Verification items for the finished model (mm, model axes). A direction names the side the tool comes from. Coordinates: 2 decimals unless noted, no trailing zeros. Write each loop counter-clockwise with the first axis right and the second up, starting at its lowest first coordinate (ties: lowest second). Pieces come first, ordered by that corner, then holes. Notation, with made-up numbers: M 82.25,74.5 L 119.25,74.5 A18 ccw 119.25,99.5 Z; hole C -33,38.25 d3. An arc over 180 degrees is marked long. Answer in a Markdown table with one row per item.
from build123d import *

# Parameters (mm, degrees)
BOSS_EXTRUDE2_DEPTH = 101.6
CUT_SWEEP2_START    = -8.197626231
CUT_SWEEP2_DEPTH    = 16.395252462


# Read off the part's stored shape, not the designer's step: Cut-Sweep2
with BuildPart() as part:
    # Sketch1 → Boss-Extrude2 (new, symmetric)
    with BuildSketch(Plane.XY):
        with BuildLine():
            Line((-50.8, 0), (-114.3, 0))
            Line((-114.3, 0), (-114.3, 12.7))
            Line((-114.3, 12.7), (-63.5, 12.7))
            ThreePointArc((-63.5, 12.7), (0, 64.757547823), (63.5, 12.7))
            Line((63.5, 12.7), (114.3, 12.7))
            Line((114.3, 12.7), (114.3, 0))
            Line((114.3, 0), (50.8, 0))
            ThreePointArc((50.8, 0), (0, 50.8), (-50.8, 0))
        make_face()
    extrude(amount=BOSS_EXTRUDE2_DEPTH, both=True)

    # Cut-Sweep2 outline → Cut-Sweep2 (cut)
    with BuildSketch(Plane.XY.offset(CUT_SWEEP2_START)):
        with BuildLine():
            Line((50.8, 0), (55.482597318, 0))
            add(Edge.make_bspline(
                [(55.482597318, 0), (55.479494195, 2.91415368), (55.255178285, 5.917770975), (54.175303072, 12.490458413), (53.25997788, 15.990881145), (50.641228247, 22.973888147), (48.970431753, 26.367184551), (44.847073202, 32.894857639), (42.443468127, 35.946208717), (37.009145884, 41.519887141), (34.016276899, 44.003484644), (27.57622226, 48.300783556), (24.203765584, 50.065786815), (13.800838479, 54.25746412), (6.656772523, 55.483587394), (-6.656785579, 55.483587394), (-13.800859436, 54.257459266), (-24.203789489, 50.065775387), (-27.576245764, 48.3007701), (-34.016297572, 44.003468622), (-37.009164361, 41.519870489), (-42.443481596, 35.946192603), (-44.847084096, 32.894842463), (-48.970437832, 26.367172857), (-50.64123252, 22.973878319), (-53.259979362, 15.990875624), (-54.175303836, 12.490454657), (-55.255178301, 5.917770093), (-55.47949419, 2.914153473), (-55.482597317, 0)],
                knots=[0.007470969, 0.007470969, 0.007470969, 0.007470969, 0.062499939, 0.062499939, 0.124999877, 0.124999877, 0.187499816, 0.187499816, 0.249999755, 0.249999755, 0.312499694, 0.312499694, 0.374999632, 0.374999632, 0.49999951, 0.49999951, 0.624999632, 0.624999632, 0.687499694, 0.687499694, 0.749999755, 0.749999755, 0.812499816, 0.812499816, 0.874999877, 0.874999877, 0.937499939, 0.937499939, 0.992529016, 0.992529016, 0.992529016, 0.992529016], degree=3))
            Line((-55.482597317, 0), (-50.8, 0))
            ThreePointArc((-50.8, 0), (0, 50.8), (50.8, 0))
        make_face()
    extrude(amount=CUT_SWEEP2_DEPTH, mode=Mode.SUBTRACT)


solid = part.part
1) Thickness scan on L1, parallel to X at y = 13, z = 43; L2, parallel to X at y = 10, z = -33.5; L3, parallel to Y at x = 76, z = -34.5. Record the ranges inside material, lowest first. Write a range as [from, to].
Response values:
| item | result |
|---|---|
| L1 | x = [-63.44, -49.11], [49.11, 63.44] |
| L2 | x = [-114.3, -49.81], [49.81, 114.3] |
| L3 | y = [0, 12.7] |
2) Release check for a two-part mould opening along X. For faces 5 (the face through (-114.3, 6, 1)), 6 (the face through (1.117, 50.788, 55.553)), 7 (the face through (-82, 0, 1)) record: +X half, -X half, draft (parallel to the pull), parting line (faces both ways), or undercut.
Response values:
| item | result |
|---|---|
| face 5 | -X half |
| face 6 | undercut |
| face 7 | draft |
3) Sectioned sample at B-B (x = -86). Record the cut outline in (y, z).
Response values:
| item | result |
|---|---|
| outline | M 0,-101.6 L 12.7,-101.6 L 12.7,101.6 L 0,101.6 Z |
4) Sectioned sample at A-A (z = 19). Record the cut outline in (x, y), then the cut area to 3 significant figures.
Response values:
| item | result |
|---|---|
| outline | M -114.3,0 L -50.8,0 A50.8 cw 50.8,0 L 114.3,0 L 114.3,12.7 L 63.5,12.7 A64.76 ccw -63.5,12.7 L -114.3,12.7 Z |
| area | 3,800 mm² |
5) Tool access check on faces 1 (the face through (-8.5, 50.5, -8.198)), 2 (the face through (83, 0, 1)), 3 (the face through (89, 12.7, 1)), 4 (the face through (-89, 12.7, 1)). Record the directions out of +Z, -Z, +X, -X, +Y, -Y that give a thin tool (end or side, any length) a straight path to the whole face; none if there is none.
Response values:
| item | result |
|---|---|
| face 1 | -Y |
| face 2 | +Z, -Z, +X, -X, -Y |
| face 3 | +Z, -Z, +X, +Y |
| face 4 | +Z, -Z, -X, +Y |
6) Depth check by flat-ended pin: pin 1 (1.5 mm diameter, centred on x = 15.5, z = -25.5, fed in from -Y); pin 2 (4 mm diameter, centred on x = -24.5, z = -20, fed in from -Y); pin 3 (1.5 mm diameter, centred on x = 38.5, z = -5.5, fed in from +Y). Enter the tip coordinate at first touch or a pass-through.
Response values:
| item | result |
|---|---|
| pin 1 | stops at y = 48.13 |
| pin 2 | stops at y = 43.34 |
| pin 3 | stops at y = 52.62 |
